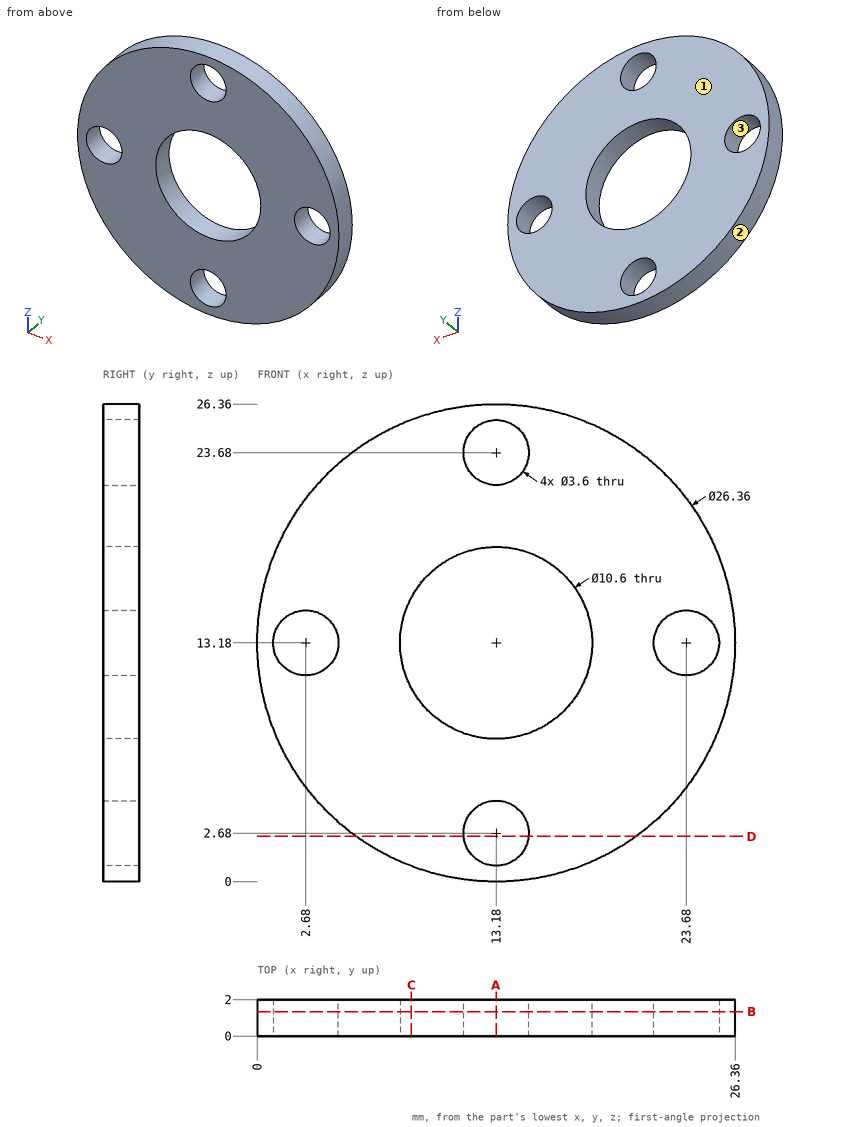
Can you work these out from the drawing? Everything is in mm from the part's minimum corner. Coordinates: 2 decimals unless noted, no trailing zeros. Order: outer loops, then holes, each group sorted by start corner. A loop starts at its lowest first (then second) coordinate and runs counter-clockwise, first axis right, second up. Notation, with made-up numbers: (37, -28.5) -> (80, -28.5) arc R15 cw to (80, -23.5) -> close; hole circle Ø8 at (69, -21). An arc over 180 degrees is marked (long way). Use one line per item in the form item = value.
Q1. Imagine slicing it at C-C, the plane x = 8.5. List the corners of the cut face in (y, z) for me, then the cut area to 3 significant figures.
From the geometry:
outline = (0, 0.86) -> (2, 0.86) -> (2, 10.69) -> (0, 10.69) -> close; (0, 15.67) -> (2, 15.67) -> (2, 25.5) -> (0, 25.5) -> close
area = 39.3 mm²
Q2. Imagine slicing it at A-A, the plane x = 13.18. List the corners of the cut face in (y, z) for me, then the cut area to 3 significant figures.
From the geometry:
outline = (0, 0) -> (2, 0) -> (2, 0.88) -> (0, 0.88) -> close; (0, 4.48) -> (2, 4.48) -> (2, 7.88) -> (0, 7.88) -> close; (0, 18.48) -> (2, 18.48) -> (2, 21.88) -> (0, 21.88) -> close; (0, 25.48) -> (2, 25.48) -> (2, 26.36) -> (0, 26.36) -> close
area = 17.1 mm²
Q3. Imagine slicing it at B-B, the plane y = 1.35. List the corners of the cut face in (x, z) for me, then the cut area to 3 significant figures.
From the geometry:
outline = circle Ø26.36 at (13.18, 13.18); hole circle Ø3.6 at (2.68, 13.18); hole circle Ø10.6 at (13.18, 13.18); hole circle Ø3.6 at (13.18, 2.68); hole circle Ø3.6 at (13.18, 23.68); hole circle Ø3.6 at (23.68, 13.18)
area = 417 mm²
Q4. I need wall thicknesses on L1, parallel to Z at x = 12.5, y = 0.8; L2, parallel to Z at x = 12.25, y = 1.9; L3, parallel to X at y = 1.2, z = 2.68. Which ranges of each line are inside material? Lowest first, please.
From the geometry:
L1 = 0.02 to 1.01, 4.35 to 7.92, 18.44 to 22.01, 25.35 to 26.34
L2 = 0.03 to 1.14, 4.22 to 7.96, 18.4 to 22.14, 25.22 to 26.33
L3 = 5.21 to 11.38, 14.98 to 21.15
Q5. Imagine slicing it at D-D, the plane z = 2.5. List the corners of the cut face in (x, y) for me.
From the geometry:
outline = (5.46, 0) -> (11.39, 0) -> (11.39, 2) -> (5.46, 2) -> close; (14.97, 0) -> (20.9, 0) -> (20.9, 2) -> (14.97, 2) -> close
Q6. We'd pull the mould along Z, two halves only. Please class the marked faces 1, 2 and 3: released by +Z, released by -Z, zero draft, split by the parting line, or undercut.
From the geometry:
face_1 = zero draft
face_2 = split by the parting line
face_3 = undercut
